from build123d import *

# Parameters (mm, degrees)
F0_W        = 31.8
F0_H        = 15.8
F1_DEPTH    = 9.6
F2_R        = 2.435
F3_DEPTH    = 1.8
F4_T        = -1.24
F5_R        = 3.2
F6_DEPTH    = 8.36
F7_T        = 1.24
F7_T3_DEPTH = 10.84
F7_T5_DEPTH = 15.8
F7_T7_DEPTH = 31.8
F9_DEPTH    = 5


# Not quite as in the source:
# - a shell that OpenCascade refuses in one call is made with other operations: the cavity is built on its own and cut out


with BuildPart() as f1:
    # F0 (on Top) → F1 (new body)
    with BuildSketch(Plane.XY):
        with Locations((15.9, 7.9)):
            Rectangle(F0_W, F0_H)
    extrude(amount=F1_DEPTH)

    # F2 (on face) → F3 (join)
    with BuildSketch(Plane.XY.offset(9.6)):
        with Locations((11.9, 11.9)):
            Circle(F2_R)
        with Locations((19.9, 11.9)):
            Circle(F2_R)
        with Locations((27.9, 11.9)):
            Circle(F2_R)
        with Locations((27.9, 3.9)):
            Circle(F2_R)
        with Locations((19.9, 3.9)):
            Circle(F2_R)
        with Locations((11.9, 3.9)):
            Circle(F2_R)
        with Locations((3.9, 3.9)):
            Circle(F2_R)
        with Locations((3.9, 11.9)):
            Circle(F2_R)
    extrude(amount=F3_DEPTH)

    # F4
    f4_openings = [f1.faces().sort_by_distance(p)[0] for p in [
        (15.9, 7.9, 0),
    ]]
    offset(amount=F4_T, openings=f4_openings, kind=Kind.INTERSECTION)

    # F5 (on face) → F6 (join, through all)
    with BuildSketch(Plane(origin=(0, 0, 8.36), x_dir=(1, 0, 0), z_dir=(0, 0, -1))):
        with Locations((7.9, -7.9)):
            Circle(F5_R)
        with Locations((15.9, -7.9)):
            Circle(F5_R)
        with Locations((23.9, -7.9)):
            Circle(F5_R)
    extrude(amount=F6_DEPTH)

    # F7: shell of thickness 1.24, made by hand


with BuildPart() as f7_core1:
    # F7_t2: copy of F1
    add(f1.part)

    # the walls: a layer under each face that stays
    f7_faces = [f7_core1.faces().sort_by_distance(p)[0] for p in [
        (0, 7.9, 4.8),
        (15.9, 15.8, 4.8),
        (15.9, 0, 4.8),
        (2.2714285714, 1.1285714286, 0),
        (15.9, 7.9, 9.6),
        (31.8, 7.9, 4.8),
        (1.24, 7.9, 4.18),
        (15.9, 14.56, 4.18),
        (30.56, 7.9, 4.18),
        (15.9, 1.24, 4.18),
        (1.465, 3.9, 10.5),
        (9.465, 3.9, 10.5),
        (17.465, 3.9, 10.5),
        (25.465, 3.9, 10.5),
        (1.465, 11.9, 10.5),
        (9.465, 11.9, 10.5),
        (17.465, 11.9, 10.5),
        (25.465, 11.9, 10.5),
        (6.1266666667, 3.46, 8.36),
        (3.9, 3.9, 11.4),
        (11.9, 3.9, 11.4),
        (19.9, 3.9, 11.4),
        (27.9, 3.9, 11.4),
        (3.9, 11.9, 11.4),
        (11.9, 11.9, 11.4),
        (19.9, 11.9, 11.4),
        (27.9, 11.9, 11.4),
        (2.705, 3.9, 9.26),
        (10.705, 3.9, 9.26),
        (18.705, 3.9, 9.26),
        (26.705, 3.9, 9.26),
        (4.7, 7.9, 4.18),
        (2.705, 11.9, 9.26),
        (10.705, 11.9, 9.26),
        (12.7, 7.9, 4.18),
        (20.7, 7.9, 4.18),
        (18.705, 11.9, 9.26),
        (26.705, 11.9, 9.26),
        (3.9, 3.9, 10.16),
        (11.9, 3.9, 10.16),
        (19.9, 3.9, 10.16),
        (27.9, 3.9, 10.16),
        (3.9, 11.9, 10.16),
        (11.9, 11.9, 10.16),
        (19.9, 11.9, 10.16),
        (27.9, 11.9, 10.16),
    ]]
    thicken(f7_faces, amount=-F7_T, mode=Mode.SUBTRACT)

    # F7_s4 → F7_t3 (cut)
    with BuildSketch(Plane.XY.offset(-1.24)):
        Polygon((1.2524, 14.5476), (0, 14.56), (0, 15.8), (1.24, 15.8), align=None)
        Polygon((1.2524, 1.2524), (0, 1.24), (0, 0), (1.24, 0), align=None)
        Polygon((30.5476, 14.5476), (30.56, 15.8), (31.8, 15.8), (31.8, 14.56), align=None)
        Polygon((30.5476, 1.2524), (31.8, 1.24), (31.8, 0), (30.56, 0), align=None)
    extrude(amount=F7_T3_DEPTH, mode=Mode.SUBTRACT)

    # F7_s6 → F7_t5 (cut)
    with BuildSketch(Plane.XZ.offset(-15.8)):
        Polygon((1.2524, 8.3476), (0, 8.36), (0, 9.6), (1.24, 9.6), align=None)
        Polygon((30.5476, 8.3476), (31.8, 8.36), (31.8, 9.6), (30.56, 9.6), align=None)
    extrude(amount=F7_T5_DEPTH, mode=Mode.SUBTRACT)

    # F7_s8 → F7_t7 (cut)
    with BuildSketch(Plane.YZ):
        Polygon((14.5476, 8.3476), (15.8, 8.36), (15.8, 9.6), (14.56, 9.6), align=None)
        Polygon((1.2524, 8.3476), (0, 8.36), (0, 9.6), (1.24, 9.6), align=None)
    extrude(amount=F7_T7_DEPTH, mode=Mode.SUBTRACT)

    # F7_s9 → F7_t10 (revolve, cut)
    with BuildSketch(Plane.XZ.offset(-3.9)):
        Polygon((6.3474, 9.6124), (6.335, 8.36), (5.095, 8.36), (5.095, 9.6), align=None)
    revolve(axis=Axis((3.9, 3.9, 9.6), (0, 0, 1)), mode=Mode.SUBTRACT)

    # F7_s11 → F7_t12 (revolve, cut)
    with BuildSketch(Plane.XZ.offset(-3.9)):
        Polygon((14.3474, 9.6124), (14.335, 8.36), (13.095, 8.36), (13.095, 9.6), align=None)
    revolve(axis=Axis((11.9, 3.9, 9.6), (0, 0, 1)), mode=Mode.SUBTRACT)

    # F7_s13 → F7_t14 (revolve, cut)
    with BuildSketch(Plane.XZ.offset(-3.9)):
        Polygon((22.3474, 9.6124), (22.335, 8.36), (21.095, 8.36), (21.095, 9.6), align=None)
    revolve(axis=Axis((19.9, 3.9, 9.6), (0, 0, 1)), mode=Mode.SUBTRACT)

    # F7_s15 → F7_t16 (revolve, cut)
    with BuildSketch(Plane.XZ.offset(-3.9)):
        Polygon((30.3474, 9.6124), (30.335, 8.36), (29.095, 8.36), (29.095, 9.6), align=None)
    revolve(axis=Axis((27.9, 3.9, 9.6), (0, 0, 1)), mode=Mode.SUBTRACT)

    # F7_s17 → F7_t18 (revolve, cut)
    with BuildSketch(Plane.XZ.offset(-11.9)):
        Polygon((6.3474, 9.6124), (6.335, 8.36), (5.095, 8.36), (5.095, 9.6), align=None)
    revolve(axis=Axis((3.9, 11.9, 9.6), (0, 0, 1)), mode=Mode.SUBTRACT)

    # F7_s19 → F7_t20 (revolve, cut)
    with BuildSketch(Plane.XZ.offset(-11.9)):
        Polygon((14.3474, 9.6124), (14.335, 8.36), (13.095, 8.36), (13.095, 9.6), align=None)
    revolve(axis=Axis((11.9, 11.9, 9.6), (0, 0, 1)), mode=Mode.SUBTRACT)

    # F7_s21 → F7_t22 (revolve, cut)
    with BuildSketch(Plane.XZ.offset(-11.9)):
        Polygon((22.3474, 9.6124), (22.335, 8.36), (21.095, 8.36), (21.095, 9.6), align=None)
    revolve(axis=Axis((19.9, 11.9, 9.6), (0, 0, 1)), mode=Mode.SUBTRACT)

    # F7_s23 → F7_t24 (revolve, cut)
    with BuildSketch(Plane.XZ.offset(-11.9)):
        Polygon((30.3474, 9.6124), (30.335, 8.36), (29.095, 8.36), (29.095, 9.6), align=None)
    revolve(axis=Axis((27.9, 11.9, 9.6), (0, 0, 1)), mode=Mode.SUBTRACT)

    # F7_s25 → F7_t26 (revolve, cut)
    with BuildSketch(Plane.XZ.offset(-7.9)):
        Polygon((11.1124, 8.3476), (11.1, 9.6), (9.86, 9.6), (9.86, 8.36), align=None)
    revolve(axis=Axis((7.9, 7.9, 8.36), (0, 0, -1)), mode=Mode.SUBTRACT)

    # F7_s27 → F7_t28 (revolve, cut)
    with BuildSketch(Plane.XZ.offset(-7.9)):
        Polygon((19.1124, 8.3476), (19.1, 9.6), (17.86, 9.6), (17.86, 8.36), align=None)
    revolve(axis=Axis((15.9, 7.9, 8.36), (0, 0, -1)), mode=Mode.SUBTRACT)

    # F7_s29 → F7_t30 (revolve, cut)
    with BuildSketch(Plane.XZ.offset(-7.9)):
        Polygon((27.1124, 8.3476), (27.1, 9.6), (25.86, 9.6), (25.86, 8.36), align=None)
    revolve(axis=Axis((23.9, 7.9, 8.36), (0, 0, -1)), mode=Mode.SUBTRACT)

    # F7_s31 → F7_t32 (revolve, cut)
    with BuildSketch(Plane.XZ.offset(-3.9)):
        Polygon((5.0826, 10.1476), (6.335, 10.16), (6.335, 11.4), (5.095, 11.4), align=None)
    revolve(axis=Axis((3.9, 3.9, 10.16), (0, 0, -1)), mode=Mode.SUBTRACT)

    # F7_s33 → F7_t34 (revolve, cut)
    with BuildSketch(Plane.XZ.offset(-3.9)):
        Polygon((13.0826, 10.1476), (14.335, 10.16), (14.335, 11.4), (13.095, 11.4), align=None)
    revolve(axis=Axis((11.9, 3.9, 10.16), (0, 0, -1)), mode=Mode.SUBTRACT)

    # F7_s35 → F7_t36 (revolve, cut)
    with BuildSketch(Plane.XZ.offset(-3.9)):
        Polygon((21.0826, 10.1476), (22.335, 10.16), (22.335, 11.4), (21.095, 11.4), align=None)
    revolve(axis=Axis((19.9, 3.9, 10.16), (0, 0, -1)), mode=Mode.SUBTRACT)

    # F7_s37 → F7_t38 (revolve, cut)
    with BuildSketch(Plane.XZ.offset(-3.9)):
        Polygon((29.0826, 10.1476), (30.335, 10.16), (30.335, 11.4), (29.095, 11.4), align=None)
    revolve(axis=Axis((27.9, 3.9, 10.16), (0, 0, -1)), mode=Mode.SUBTRACT)

    # F7_s39 → F7_t40 (revolve, cut)
    with BuildSketch(Plane.XZ.offset(-11.9)):
        Polygon((5.0826, 10.1476), (6.335, 10.16), (6.335, 11.4), (5.095, 11.4), align=None)
    revolve(axis=Axis((3.9, 11.9, 10.16), (0, 0, -1)), mode=Mode.SUBTRACT)

    # F7_s41 → F7_t42 (revolve, cut)
    with BuildSketch(Plane.XZ.offset(-11.9)):
        Polygon((13.0826, 10.1476), (14.335, 10.16), (14.335, 11.4), (13.095, 11.4), align=None)
    revolve(axis=Axis((11.9, 11.9, 10.16), (0, 0, -1)), mode=Mode.SUBTRACT)

    # F7_s43 → F7_t44 (revolve, cut)
    with BuildSketch(Plane.XZ.offset(-11.9)):
        Polygon((21.0826, 10.1476), (22.335, 10.16), (22.335, 11.4), (21.095, 11.4), align=None)
    revolve(axis=Axis((19.9, 11.9, 10.16), (0, 0, -1)), mode=Mode.SUBTRACT)

    # F7_s45 → F7_t46 (revolve, cut)
    with BuildSketch(Plane.XZ.offset(-11.9)):
        Polygon((29.0826, 10.1476), (30.335, 10.16), (30.335, 11.4), (29.095, 11.4), align=None)
    revolve(axis=Axis((27.9, 11.9, 10.16), (0, 0, -1)), mode=Mode.SUBTRACT)


with BuildPart() as f1_1:
    add(f1.part)

    # what is left inside the walls is the cavity
    f7_cavity = [f7_core1.part.solids().sort_by_distance(p)[0] for p in [
        (5.9524, 7.9, 2.786667),
        (13.9524, 7.9, 2.786667),
        (21.9524, 7.9, 2.786667),
    ]]
    add(f7_cavity, mode=Mode.SUBTRACT)

    # F8 (on face) → F9 (join)
    with BuildSketch(Plane(origin=(0, 0, 8.36), x_dir=(1, 0, 0), z_dir=(0, 0, -1))):
        with BuildLine():
            Line((16.4, -1.24), (15.4, -1.24))
            Line((15.4, -1.24), (15.4, -4.7393038741))
            ThreePointArc((15.4, -4.7393038741), (15.9, -4.7), (16.4, -4.7393038741))
            Line((16.4, -4.7393038741), (16.4, -1.24))
        make_face()
        with BuildLine():
            ThreePointArc((16.4, -11.0606961259), (15.9, -11.1), (15.4, -11.0606961259))
            Line((15.4, -11.0606961259), (15.4, -14.56))
            Line((15.4, -14.56), (16.4, -14.56))
            Line((16.4, -14.56), (16.4, -11.0606961259))
        make_face()
    extrude(amount=F9_DEPTH)


solid = f1_1.part
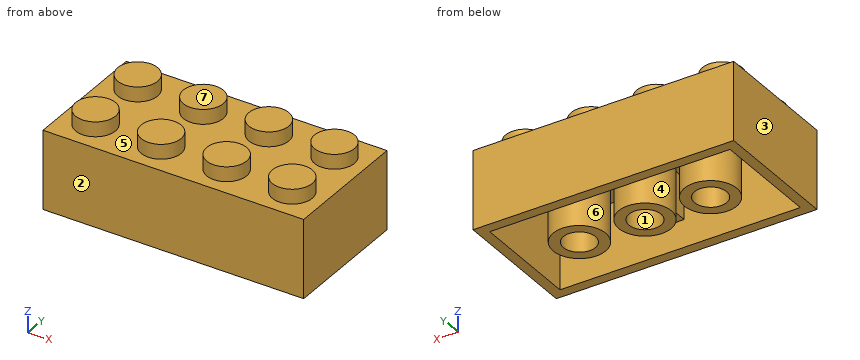
Part model, mm, in its own coordinate system. Face numbers are marked on the shaded views. A direction names the side the tool comes from. Give positions to 0.01 mm unless a question says otherwise; leave off trailing zeros. Order: outer loops, then holes, each group sorted by start corner. A loop starts at its lowest first (then second) coordinate and runs counter-clockwise, first axis right, second up. Notation, with made-up numbers: (84, 17) - (126, 17) arc R25 ccw to (126, 51) - close; hole circle Ø7 at (55, 88.25). An arc over 180 degrees is marked (long way). One line per question, with ' | ' between items.
1. Which spindle directions (+Z, -Z, +X, -X, +Y, -Y) get a long thin tool onto all of the face, cutting with end or side? Do the marked faces 5, 6 and 7. Say none if no direction does.
Filled in:
face 5: +Z | face 6: -Z | face 7: +Z, +X, -X, +Y, -Y
2. Drop flat-ended pins along their axis: P1, Ø1.2, axis at x = 24, y = 8, coming from the -Z side; P2, Ø0.7, axis at x = 19.5, y = 3.5, coming from the -Z side. Give the stop position or say it passes through.
Filled in:
P1: z = 8.36 | P2: z = 10.16
3. Band-saw the part on C-C on x = 7.9. List the corners of the cut face in (y, z).
Filled in:
outline: (0, 0) - (1.24, 0) - (1.24, 8.36) - (4.7, 8.36) - (4.7, 0) - (5.94, 0) - (5.94, 8.36) - (9.86, 8.36) - (9.86, 0) - (11.1, 0) - (11.1, 8.36) - (14.56, 8.36) - (14.56, 0) - (15.8, 0) - (15.8, 9.6) - (0, 9.6) - close
4. Band-saw the part on B-B on z = 3. List the corners of the cut face in (x, y).
Filled in:
outline: (0, 0) - (31.8, 0) - (31.8, 15.8) - (0, 15.8) - close; circle Ø6.4 at (7.9, 7.9); circle Ø6.4 at (15.9, 7.9); circle Ø6.4 at (23.9, 7.9); hole (1.24, 1.24) - (30.56, 1.24) - (30.56, 14.56) - (1.24, 14.56) - close; hole circle Ø3.92 at (7.9, 7.9); hole circle Ø3.92 at (15.9, 7.9); hole circle Ø3.92 at (23.9, 7.9)
5. Drill centre lines: probe 1 along X at (y, z) = (14, 7.25); probe 2 along X at (y, z) = (3.9, 9.3) (3 decimals); probe 3 along Y at (x, z) = (11.9, 9) (3 decimals). Where is each one in solid material? Low to high.
Filled in:
probe 1: 0 to 1.24, 15.4 to 16.4, 30.56 to 31.8 | probe 2: 0 to 2.705, 5.095 to 10.705, 13.095 to 18.705, 21.095 to 26.705, 29.095 to 31.8 | probe 3: 0 to 2.705, 5.095 to 10.705, 13.095 to 15.8
6. Pull direction X, two halves, no side cores. Call the marked faces 1, 2, 3 and 4: +X half, -X half, draft (parallel to the pull), parting line (faces both ways), or undercut.
Filled in:
face 1: undercut | face 2: draft | face 3: -X half | face 4: undercut
7. Band-saw the part on D-D on y = 14. List the corners of the cut face in (x, z), then the cut area to 3 significant figures.
Filled in:
outline: (0, 0) - (1.24, 0) - (1.24, 8.36) - (15.4, 8.36) - (15.4, 3.36) - (16.4, 3.36) - (16.4, 8.36) - (30.56, 8.36) - (30.56, 0) - (31.8, 0) - (31.8, 9.6) - (29.13, 9.6) - (29.13, 11.4) - (26.67, 11.4) - (26.67, 9.6) - (21.13, 9.6) - (21.13, 11.4) - (18.67, 11.4) - (18.67, 9.6) - (13.13, 9.6) - (13.13, 11.4) - (10.67, 11.4) - (10.67, 9.6) - (5.13, 9.6) - (5.13, 11.4) - (2.67, 11.4) - (2.67, 9.6) - (0, 9.6) - close | area: 82.9 mm²
8. Band-saw the part on A-A on z = 5. List the corners of the cut face in (x, y), then the cut area to 3 significant figures.
Filled in:
outline: (0, 0) - (31.8, 0) - (31.8, 15.8) - (0, 15.8) - close; circle Ø6.4 at (7.9, 7.9); circle Ø6.4 at (23.9, 7.9); hole (1.24, 1.24) - (15.4, 1.24) - (15.4, 4.74) arc R3.2 cw to (15.4, 11.06) - (15.4, 14.56) - (1.24, 14.56) - close; hole circle Ø3.92 at (7.9, 7.9); hole circle Ø3.92 at (15.9, 7.9); hole (16.4, 1.24) - (30.56, 1.24) - (30.56, 14.56) - (16.4, 14.56) - (16.4, 11.06) arc R3.2 cw to (16.4, 4.74) - close; hole circle Ø3.92 at (23.9, 7.9) | area: 179 mm²
